The listing builds one solid part. Answer for the finished solid, in the listing's coordinates (mm). A direction names the side the tool comes from. Give positions to 0.01 mm unless a question says otherwise; leave off trailing zeros. Loops run counter-clockwise (first coordinate to the right, second up) from the corner with the lowest first, then second, coordinate; pieces in that order, holes last. Notation, with made-up numbers: M -21,-38 L 25,-38 A20 cw 25,-24 Z; hole C -10,-15.5 d3. An arc over 180 degrees is marked long. Use one line per item in the form item = value. Start each with the question number.
1. For faces 4 (the face through (41.91, -119.597, 1.84)), 5 (the face through (-39.4, -245.1, 1.8)), 6 (the face through (-58.05, -216.65, 1.79)), determine the directions among +Z, -Z, +X, -X, +Y, -Y from which every point of the face is accessible in a straight line to the end or side of a thin tool.
2. Each of these flat-tipped pins is pushed along its axis until it touches: pin 1 Ø1.1 at (y, z) = (-255, 2) entering from -X; pin 2 Ø1.8 at (y, z) = (-161, 2) entering from +X; pin 3 Ø1.5 at (x, z) = (33.5, 1.5) entering from -Y. Where does it stop, or does it pass through?
3. The part is cut by section D-D (y = -126.5). Write down the section's boundary in (x, z), and give its area (3 significant figures).
4. The mould has two halves that part along X. Classify faces 1 (the face through (58.626, -218.796, 1.789)), 2 (the face through (3, -165, 0)), 3 (the face through (-17.93, -95.78, 1.79)): released by +X, released by -X, zero draft, split by the parting line, or undercut.
5. The part is cut by section A-A (y = -94.56). Write down the section's boundary in (x, z) (3 decimals), and give its area (3 significant figures).
6. The part is cut by section B-B (y = -217). Write down the section's boundary in (x, z), and give its area (3 significant figures).
7. The part is cut by section C-C (y = -182). Write down the section's boundary in (x, z).
8. Straight lines are drawn through the part: line 1 (X direction, y = -238, z = 1); line 2 (X direction, y = -273.5, z = 0.95); line 3 (X direction, y = -103, z = 0.35). For each, find the intervals that lie inside material, in ascending order. Write a range as from..to.
from build123d import *

# Parameters (mm, degrees)
BOSS_EXTRUDE2_DEPTH = 3.628571429
FILLET1_R           = 25
BOSS_EXTRUDE4_DEPTH = 3.628571429
CUT_EXTRUDE2_DEPTH  = 336.434355024
CIRPATTERN8_COUNT   = 20
CIRPATTERN8_ANGLE   = 28.5
SKETCH5_R           = 3.175
CUT_EXTRUDE3_DEPTH  = 338.743409804
SKETCH17_R          = 3.175
CUT_EXTRUDE4_DEPTH  = 338.743409804


with BuildPart() as part:
    # Sketch3 → Boss-Extrude2 (new body)
    with BuildSketch(Plane.XY):
        with BuildLine():
            Line((-140, -79.56), (-140, -109.56))
            Line((-140, -109.56), (-29.356513523, -109.56))
            Line((-29.356513523, -109.56), (-78.888044947, -294.414191853))
            ThreePointArc((-78.888044947, -294.414191853), (0, -304.8), (78.888044947, -294.414191853))
            Line((78.888044947, -294.414191853), (29.356513523, -109.56))
            Line((29.356513523, -109.56), (140, -109.56))
            Line((140, -109.56), (140, -79.56))
            Line((140, -79.56), (-140, -79.56))
        make_face()
    extrude(amount=BOSS_EXTRUDE2_DEPTH)

    # Fillet1
    fillet1_edges = [part.edges().sort_by_distance(p)[0] for p in [
        (29.356513523, -109.56, 1.814285714),
        (-29.356513523, -109.56, 1.814285714),
    ]]
    fillet(fillet1_edges, radius=FILLET1_R)

    # Sketch14 → Boss-Extrude4 (add)
    with BuildSketch(Plane(origin=(0, 0, 0), x_dir=(-1, 0, 0), z_dir=(0, 0, -1))):
        with BuildLine():
            Line((78.910933272, -297.036934084), (78.888044947, -294.414191853))
            ThreePointArc((78.888044947, -294.414191853), (76.959432674, -294.924203351), (75.027523715, -295.421581279))
            Line((75.027523715, -295.421581279), (76.289081309, -297.721097125))
            Line((76.289081309, -297.721097125), (78.910933272, -297.036934084))
        make_face()
    boss_extrude4 = extrude(amount=-BOSS_EXTRUDE4_DEPTH)

    # Sketch16 → Cut-Extrude2 (cut, symmetric)
    with BuildSketch(Plane(origin=(0, 0, 0), x_dir=(-1, 0, 0), z_dir=(0, 0, -1))):
        Polygon((372.937709596, -838.440145613), (75.027523715, -295.421581279), (73.765262731, -293.12078332), (71.19993834, -293.754449124), (71.154137831, -296.378353915), (60.344615656, -915.654378233), (357.400151379, -2118.250141136), (669.993245319, -2041.035908516), align=None)
    cut_extrude2 = extrude(amount=CUT_EXTRUDE2_DEPTH, both=True, mode=Mode.SUBTRACT)

    # CirPattern8: Boss-Extrude4, Cut-Extrude2 ×20 about axis
    cirpattern8_axis = Axis((0, 0, 0), (0, 0, 1))
    add([boss_extrude4.rotate(cirpattern8_axis, i * CIRPATTERN8_ANGLE / (CIRPATTERN8_COUNT - 1)) for i in range(1, CIRPATTERN8_COUNT)])
    add([cut_extrude2.rotate(cirpattern8_axis, i * CIRPATTERN8_ANGLE / (CIRPATTERN8_COUNT - 1)) for i in range(1, CIRPATTERN8_COUNT)], mode=Mode.SUBTRACT)

    # Sketch5 → Cut-Extrude3 (cut, through all)
    with BuildSketch(Plane(origin=(0, 0, 0), x_dir=(-1, 0, 0), z_dir=(0, 0, -1))):
        with Locations((-15, -94.56)):
            Circle(SKETCH5_R)
        with Locations((15, -94.56)):
            Circle(SKETCH5_R)
        with BuildLine():
            Line((-123.5, -94.56), (-123.5, -100.91))
            ThreePointArc((-123.5, -100.91), (-120, -104.41), (-116.5, -100.91))
            Line((-116.5, -100.91), (-116.5, -94.56))
            Line((-116.5, -94.56), (-116.5, -88.21))
            ThreePointArc((-116.5, -88.21), (-120, -84.71), (-123.5, -88.21))
            Line((-123.5, -88.21), (-123.5, -94.56))
        make_face()
        with BuildLine():
            Line((116.5, -94.56), (116.5, -88.21))
            ThreePointArc((116.5, -88.21), (120, -84.71), (123.5, -88.21))
            Line((123.5, -88.21), (123.5, -94.56))
            Line((123.5, -94.56), (123.5, -100.91))
            ThreePointArc((123.5, -100.91), (120, -104.41), (116.5, -100.91))
            Line((116.5, -100.91), (116.5, -94.56))
        make_face()
    extrude(amount=-CUT_EXTRUDE3_DEPTH, mode=Mode.SUBTRACT)

    # Sketch17 → Cut-Extrude4 (cut, through all)
    with BuildSketch(Plane(origin=(0, 0, 0), x_dir=(-1, 0, 0), z_dir=(0, 0, -1))):
        Polygon((-28.711660115, -141.33134449), (-64.419853025, -277.589898046), (-15, -213.409642912), align=None)
        Polygon((15, -213.409642912), (64.419853025, -277.589898046), (28.711660115, -141.33134449), align=None)
        with BuildLine():
            Line((57.677925946, -286.294618468), (59.356743472, -285.913498464))
            Line((59.356743472, -285.913498464), (5, -223.409642912))
            Line((5, -223.409642912), (5, -292.259285824))
            ThreePointArc((5, -292.259285824), (31.480548191, -290.527384931), (57.677925946, -286.294618468))
        make_face()
        with BuildLine():
            Line((-5, -223.409642912), (-59.372890863, -285.932066063))
            ThreePointArc((-59.372890863, -285.932066063), (-32.341547535, -290.428544105), (-5, -292.259285824))
            Line((-5, -292.259285824), (-5, -223.409642912))
        make_face()
        Polygon((5, -203.409642912), (19.937147844, -134.56), (5, -134.56), align=None)
        Polygon((-19.937147844, -134.56), (-5, -203.409642912), (-5, -134.56), align=None)
        with Locations((0, -193.697232184)):
            Circle(SKETCH17_R)
        with Locations((0, -154.272410728)):
            Circle(SKETCH17_R)
        with Locations((0, -233.12205364)):
            Circle(SKETCH17_R)
        with Locations((0, -272.546875096)):
            Circle(SKETCH17_R)
        with Locations((71.194365296, -284.361242536)):
            Circle(SKETCH17_R)
        with Locations((-71.194365296, -284.361242536)):
            Circle(SKETCH17_R)
    extrude(amount=-CUT_EXTRUDE4_DEPTH, mode=Mode.SUBTRACT)


solid = part.part
Derived:
q1.face_4 = +Z, -Z, +X
q1.face_5 = +Z, -Z
q1.face_6 = +Z, -Z, -X
q2.pin_1 = -68.47
q2.pin_2 = 43.38
q2.pin_3 = -305.59
q3.outline = M -38.27,0 L 38.27,0 L 38.27,3.63 L -38.27,3.63 Z
q3.area = 278 mm2
q4.face_1 = released by +X
q4.face_2 = zero draft
q4.face_3 = undercut
q5.outline = M -140,0 L -123.5,0 L -123.5,3.629 L -140,3.629 Z; M -116.5,0 L -18.175,0 L -18.175,3.629 L -116.5,3.629 Z; M -11.825,0 L 11.825,0 L 11.825,3.629 L -11.825,3.629 Z; M 18.175,0 L 116.5,0 L 116.5,3.629 L 18.175,3.629 Z; M 123.5,0 L 140,0 L 140,3.629 L 123.5,3.629 Z
q5.area = 919 mm2
q6.outline = M -58.14,0 L -48.54,0 L -48.54,3.63 L -58.14,3.63 Z; M -17.76,0 L 17.76,0 L 17.76,3.63 L -17.76,3.63 Z; M 48.54,0 L 58.14,0 L 58.14,3.63 L 48.54,3.63 Z
q6.area = 199 mm2
q7.outline = M -48.77,0 L -39.37,0 L -39.37,3.63 L -48.77,3.63 Z; M -20.98,0 L -9.64,0 L -9.64,3.63 L -20.98,3.63 Z; M -5,0 L 5,0 L 5,3.63 L -5,3.63 Z; M 9.64,0 L 20.98,0 L 20.98,3.63 L 9.64,3.63 Z; M 39.37,0 L 48.77,0 L 48.77,3.63 L 39.37,3.63 Z
q8.line_1 = -63.77..-54.04, -33.93..-17.69, -5..5, 17.69..33.93, 54.04..63.77
q8.line_2 = -73.28..-63.35, -61.27..-48.56, -5..-3.03, 3.03..5, 48.56..61.27, 63.35..73.28
q8.line_3 = -140..-122.81, -117.19..117.19, 122.81..140
